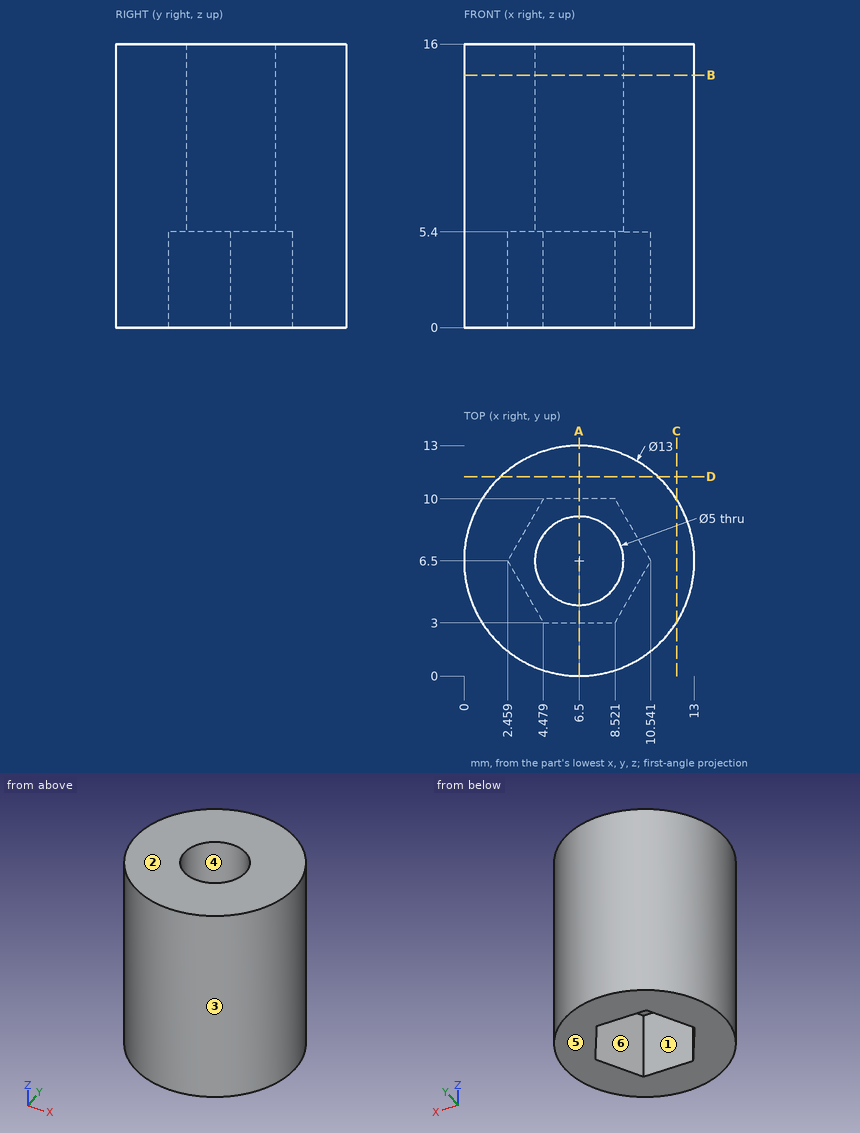
Design review of the part shown in the three views and the two pictorial views. Dimensions are in mm from the part's minimum x, y and z. A direction names the side the tool comes from. Coordinates: 2 decimals unless noted, no trailing zeros. Write each loop counter-clockwise with the first axis right and the second up, starting at its lowest first coordinate (ties: lowest second). Pieces come first, ordered by that corner, then holes. Notation, with made-up numbers: (85.5, 22.5) -> (127.5, 22.5) arc R17 ccw to (127.5, 30.5) -> close; hole circle Ø8 at (-21, 57). An arc over 180 degrees is marked (long way). Answer in a Markdown table with one row per item.
1. Wall thickness on probe 1 along Y at (x, z) = (6.5, 9); probe 2 along Y at (x, z) = (0.5, 9.25) (1 decimal); probe 3 along Z at (x, y) = (9, 4.75): over which ranges is each line inside the solid? List them lowest first. Write a range as [from, to].
Answers below:
| item | result |
|---|---|
| probe 1 | y = [0, 4], [9, 13] |
| probe 2 | y = [4, 9] |
| probe 3 | z = [5.4, 16] |
2. We need section C-C, the plane x = 12. State the section outline as (y, z) points (1 decimal), and give its area (3 significant figures).
Answers below:
| item | result |
|---|---|
| outline | (3, 0) -> (10, 0) -> (10, 16) -> (3, 16) -> close |
| area | 111 mm^2 |
3. We need section B-B, the plane z = 14.25. State the section outline as (x, y) points.
Answers below:
| item | result |
|---|---|
| outline | circle Ø13 at (6.5, 6.5); hole circle Ø5 at (6.5, 6.5) |
4. We need section D-D, the plane y = 11.25. State the section outline as (x, z) points.
Answers below:
| item | result |
|---|---|
| outline | (2.06, 0) -> (10.94, 0) -> (10.94, 16) -> (2.06, 16) -> close |
5. Draft analysis for pull direction X (two halves, no side actions). For the marked faces 3, 4, 5 and 6, state which applies: +X half, -X half, draft (parallel to the pull), parting line (faces both ways), or undercut.
Answers below:
| item | result |
|---|---|
| face 3 | parting line |
| face 4 | undercut |
| face 5 | draft |
| face 6 | undercut |
6. Clearance check with flat-ended pins moving along their axes: pin 1 Ø1 at (x, z) = (8, 8) entering from +Y; pin 2 Ø3 at (x, y) = (6.5, 6.5) entering from -Z; pin 3 Ø2 at (x, y) = (4.5, 7) entering from -Z; pin 4 Ø5 at (x, z) = (5, 5.5) entering from +Y. State where each tip first meets the part, or that it passes through.
Answers below:
| item | result |
|---|---|
| pin 1 | stops at y = 12.92 |
| pin 2 | passes through |
| pin 3 | stops at z = 5.4 |
| pin 4 | stops at y = 13 |
7. For the marked faces 1 and 2, list the 3-axis set-ups (+Z, -Z, +X, -X, +Y, -Y) from which the entire face can be reached by the end or side of a thin tool; tool diameter is ignored.
Answers below:
| item | result |
|---|---|
| face 1 | -Z |
| face 2 | +Z, +X, -X, +Y, -Y |
8. We need section A-A, the plane x = 6.5. State the section outline as (y, z) points, and give its area (3 significant figures).
Answers below:
| item | result |
|---|---|
| outline | (0, 0) -> (3, 0) -> (3, 5.4) -> (4, 5.4) -> (4, 16) -> (0, 16) -> close; (9, 5.4) -> (10, 5.4) -> (10, 0) -> (13, 0) -> (13, 16) -> (9, 16) -> close |
| area | 117 mm^2 |
